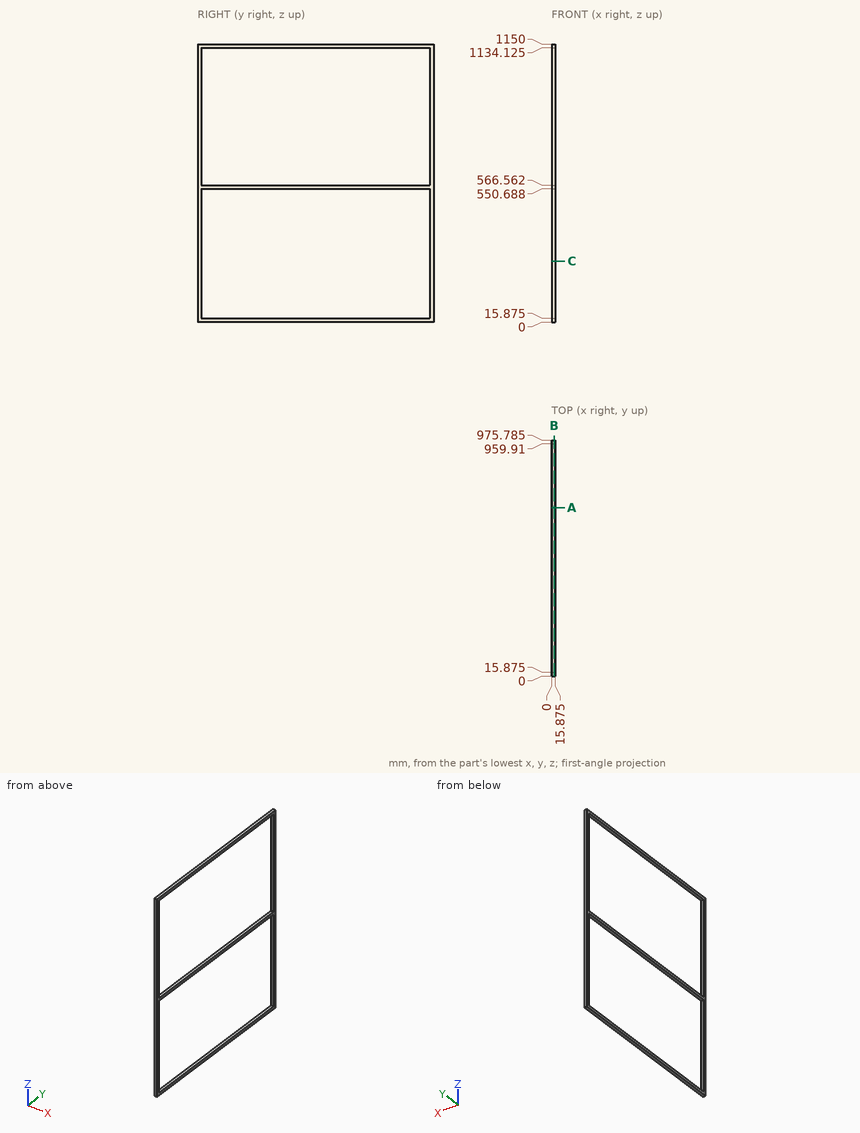
Check sheet for the drawn part. Datum: minimum x, y, z corner. Units: mm. Give positions to 0.01 mm unless a question says otherwise; leave off trailing zeros. Order: outer loops, then holes, each group sorted by start corner. A loop starts at its lowest first (then second) coordinate and runs counter-clockwise, first axis right, second up. Notation, with made-up numbers: (-14, -27) - (36, -27) arc R11 cw to (36, -19) - close; hole circle Ø3 at (62, 70.25). An arc over 180 degrees is marked (long way). Answer in a Markdown table with one row per item. Add a question column.
Q1. Material ranges on probe 1 along Z at (x, y) = (3.75, 299) (1 decimal); probe 2 along Y at (x, z) = (15.25, 276) (1 decimal), recorded low to high. Write a range as from..to.
Q2. Cross-section at A-A, the plane y = 696. Enter the section's corners in (x, z) (1 decimal).
Q3. Gauge pin test, flat end, axial feed: pin 1 (5 mm diameter, centred on x = 11, z = 303.5, fed in from -Y). Record the tip position at first contact, or that the pin passes through.
Q4. Cross-section at B-B, the plane x = 10.5. Enter the section's corners in (y, z) (1 decimal).
Q5. Cross-section at C-C, the plane z = 252.5. Enter the section's corners in (x, y) (1 decimal), then the cut area to 3 significant figures.
Check values:
| question | item | result |
|---|---|---|
| 1 | probe 1 | z = 0..15.9, 550.7..566.6, 1134.1..1150 |
| 1 | probe 2 | y = 0..15.9, 959.9..975.8 |
| 2 | outline | (0, 0) - (15.9, 0) - (15.9, 15.9) - (0, 15.9) - close; (0, 550.7) - (15.9, 550.7) - (15.9, 566.6) - (0, 566.6) - close; (0, 1134.1) - (15.9, 1134.1) - (15.9, 1150) - (0, 1150) - close |
| 3 | pin 1 | stops at y = 0 |
| 4 | outline | (0, 0) - (975.8, 0) - (975.8, 1150) - (0, 1150) - close; hole (15.9, 15.9) - (959.9, 15.9) - (959.9, 550.7) - (15.9, 550.7) - close; hole (15.9, 566.6) - (959.9, 566.6) - (959.9, 1134.1) - (15.9, 1134.1) - close |
| 5 | outline | (0, 0) - (15.9, 0) - (15.9, 15.9) - (0, 15.9) - close; (0, 959.9) - (15.9, 959.9) - (15.9, 975.8) - (0, 975.8) - close |
| 5 | area | 504 mm^2 |
